The drawing under review shows one solid part. Ordinate dimensions are in mm from its lowest x, y, z. Give positions to 0.01 mm unless a question says otherwise; leave off trailing zeros. Order: outer loops, then holes, each group sorted by start corner. A loop starts at its lowest first (then second) coordinate and runs counter-clockwise, first axis right, second up. Notation, with made-up numbers: (-38, 0.5) -> (16, 0.5) arc R28 cw to (16, 21.5) -> close; hole circle Ø9 at (-14, 10). An arc over 180 degrees is marked (long way). One line per item, written item: value.
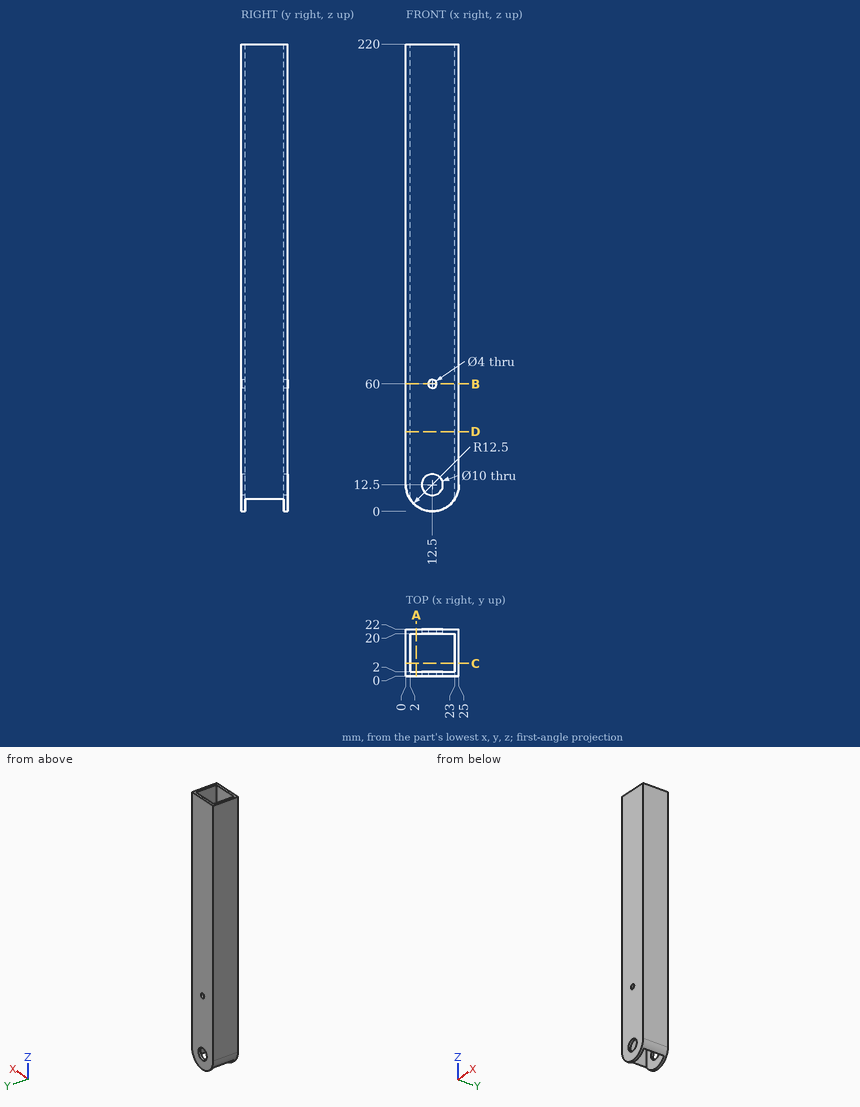
Item 1: Add section A-A on x = 5. Give the boundary of the cut face in (y, z).
Returned:
outline: (0, 2.5) -> (2, 2.5) -> (2, 220) -> (0, 220) -> close; (20, 2.5) -> (22, 2.5) -> (22, 220) -> (20, 220) -> close
Item 2: Add section B-B on z = 60. Give the boundary of the cut face in (x, y), plus the area to 3 significant figures.
Returned:
outline: (0, 0) -> (10.5, 0) -> (10.5, 2) -> (2, 2) -> (2, 20) -> (10.5, 20) -> (10.5, 22) -> (0, 22) -> close; (14.5, 0) -> (25, 0) -> (25, 22) -> (14.5, 22) -> (14.5, 20) -> (23, 20) -> (23, 2) -> (14.5, 2) -> close
area: 156 mm²
Item 3: Add section D-D on z = 37.5. Give the boundary of the cut face in (x, y), plus the area to 3 significant figures.
Returned:
outline: (0, 0) -> (25, 0) -> (25, 22) -> (0, 22) -> close; hole (2, 2) -> (23, 2) -> (23, 20) -> (2, 20) -> close
area: 172 mm²
Item 4: To check wall thickness, follow line 1 along Z through (x, y) = (12.5, 21.45); line 2 along Y through (x, z) = (3.25, 48); line 3 along X through (y, z) = (5, 66.5). State the ranges of each line that lie inside material, in increasing order. Write a range as from..to.
Returned:
line 1: 0..7.5, 17.5..58, 62..220
line 2: 0..2, 20..22
line 3: 0..2, 23..25
Item 5: Add section C-C on y = 6. Give the boundary of the cut face in (x, z), plus the area to 3 significant figures.
Returned:
outline: (0, 12.5) arc R12.5 ccw to (2, 5.72) -> (2, 220) -> (0, 220) -> close; (23, 5.72) arc R12.5 ccw to (25, 12.5) -> (25, 220) -> (23, 220) -> close
area: 848 mm²
